Autodesk Inventor part; units mm, degrees
ref_plane "Work Plane1" through (29, 0, 0) normal (0, -1, 0) x (1, 0, 0)
ref_plane "YZ Plane" through (0, 0, 0) normal (1, 0, 0) x (0, 1, 0)
ref_plane "XZ Plane" through (0, 0, 0) normal (0, 1, 0) x (-1, 0, 0)
sketch "Rascunho1" plane through (0, 0, 0) normal (0, 0, 1) x (1, 0, 0)
  line L0 (-2.6667, 0) -> (120, 0)
  line L1 (120, 0) -> (120, 6)
  line L2 (120, 6) -> (5, 6)
  line L3 (5, 6) -> (3.9264, 6)
  line L4 (3.9264, 6) -> (0, 6)
  line L5 (0, 6) -> (0, 9)
  line L6 (0, 9) -> (-12, 9)
  line L7 (-12, 9) -> (-12, 5.7735)
  line L8 (-12, 5.7735) -> (-6, 5.7735)
  line L9 (-6, 5.7735) -> (-2.6667, 0)
  line L10 (-38.4, 0) -> (146.4, 0)
  line L11 (0, -1.8) -> (0, 10.8)
  line L12 (5, 6) -> (0, 6) construction
  dimension "d1" = 115
  dimension "d2" = 1.0736
  dimension "d3" = 12
  dimension "d4" = 6
  dimension "d5" = 60
  dimension "d6" = 12
  dimension "d7" = 12
  dimension "d8" = 11.547
  dimension "d9" = 18
  dimension "d26" = 120
revolve "Corpo" add sketch "Rascunho1" angle 360 about axis through (-2.6667, 0, 0) along (1, 0, 0)
sketch "Rascunho2" plane through (-12, 0, 0) normal (-1, 0, 0) x (0, 0, 1)
  circle A0 centre (0, 0) radius 5.7735
  line L0 (0, -12.6) -> (0, 12.6)
  line L1 (-12.6, 0) -> (12.6, 0)
  line L2 (5.7735, 0) -> (2.8868, -5)
  line L3 (2.8868, -5) -> (-2.8868, -5)
  line L4 (-2.8868, -5) -> (-5.7735, 0)
  line L5 (-5.7735, 0) -> (-2.8868, 5)
  line L6 (-2.8868, 5) -> (2.8868, 5)
  line L7 (2.8868, 5) -> (5.7735, 0)
extrude "Fenda" add sketch "Rascunho2" against normal up to next contours L7 A0 | A0 L2 | L6 L0 A0 | A0 L0 L3 | L0 L6 A0 | A0 L3 L0 | L4 A0 | A0 L5
fillet "Raio de arredondamento1" radius 1.2 1 edges at (-12, -9, 0)
thread "Rosca"
chamfer "Chanfrar1" distance 1.0735 distance2 1.0735 1 edges at (120, -6, 0) measured on face at (120, 1.668, 0.0818)
ref_plane "Work Plane1" through (29, 0, 0) normal (0, -1, 0) x (1, 0, 0)
fillet "Fillet2" radius 0.1 1 edges at (0, -6, 0)
fillet "Fillet3" radius 14 1 edges at (120, -4.9265, 0)
equation "\"d1\" = GEL"
equation "\"d3\" = KOH"
equation "\"d4\" = INTI"
equation "\"d6\" = GD"
equation "\"d7\" = BDM"
equation "\"d8\" = 1.1547 * SW"
equation "\"d9\" = KOD"
equation "\"d26\" = NLG"
equation "\"d17\" = RR"
equation "\"d13\" = GEL"
equation "\"d15\" = -0.5 * SPD + 0.5 * GD"
equation "\"d16\" = GUL"
equation "\"d30\" = R"
equation "\"GD\" = NND"
equation "\"NLG\" = 120"
equation "\"GEL\" = 115"
equation "\"KOD\" = 18"
equation "\"KOH\" = 12"
equation "\"INTI\" = 6"
equation "\"GAL\" = 0.61345 * PTC"
equation "\"GUL\" = 0.61345 * PTC"
equation "\"BDM\" = NND"
equation "\"RR\" = 1.2"
equation "\"SPD\" = NND - 1.2269 * PTC"
equation "\"R\" = 0.1"
equation "\"TOA\" = 30deg"
equation "\"GD1\" = THREADDIA - 1.2269 * PTC"
equation "\"THREADDIA\" = 12"
equation "\"FAWI\" = 45deg"
equation "\"ANG\" = 120deg"
equation "\"PTC\" = 1.75"
equation "\"NND\" = 12"
equation "\"E0\" = 1.155 * SW"
properties part number "DIN 912 - M12x120" material "Aço Inox AISI 304"
For this review, take the finished solid that the model builds, in its own axes (mm). A direction names the side the tool comes from. Give positions to 0.01 mm unless a question says otherwise; leave off trailing zeros. Answer in a Markdown table with one row per item. Add a question column.
(1) For pin 1 (10 mm diameter, centred on x = 25.5, z = 6, fed in from -Y); pin 2 (1.5 mm diameter, centred on y = -7, z = 6, fed in from +X); pin 3 (8 mm diameter, centred on x = 56.5, y = 2.5, fed in from -Z), all flat-tipped, find the tip position at first contact; note any pin that passes through.
(2) Wall thickness on probe 1 along X at (y, z) = (-5.5, -5); probe 2 along Y at (x, z) = (-6, -3); probe 3 along X at (y, z) = (-2.75, 8.25): over which ranges is each line inside the solid? List them lowest first. Write a range as [from, to].
(3) Mouldability with a two-part tool opening along Z and no side actions: class faces 1 (the face through (-5.476, -1.172, -8.923)), 2 (the face through (0, 2, -6)), 3 (the face through (-9, -5, 0)), 4 (the face through (-2.875, 0.344, -0.108)) as +Z half, -Z half, draft (parallel to the pull), parting line (faces both ways), or undercut.
(4) For faces 5 (the face through (-8.822, 2.535, 4.31)), 6 (the face through (-12, -2, 5)), 7 (the face through (59, -6, 0)), list the 3-axis set-ups (+Z, -Z, +X, -X, +Y, -Y) from which the entire face can be reached by the end or side of a thin tool; tool diameter is ignored.
Evaluation:
| question | item | result |
|---|---|---|
| 1 | pin 1 | stops at y = -5.92 |
| 1 | pin 2 | stops at x = 0 |
| 1 | pin 3 | stops at z = -6 |
| 2 | probe 1 | x = [-12, 0] |
| 2 | probe 2 | y = [-8.49, -4.8], [4.8, 8.49] |
| 2 | probe 3 | x = [-11.6, 0] |
| 3 | face 1 | parting line |
| 3 | face 2 | draft |
| 3 | face 3 | undercut |
| 3 | face 4 | undercut |
| 4 | face 5 | -X |
| 4 | face 6 | +Z, -Z, -X, +Y, -Y |
| 4 | face 7 | +X |
